The listing builds one solid part. Answer for the finished solid, in the listing's coordinates (mm). A direction names the side the tool comes from. Coordinates: 2 decimals unless noted, no trailing zeros. Write each loop counter-clockwise with the first axis right and the second up, starting at its lowest first coordinate (ties: lowest second). Pieces come first, ordered by that corner, then holes. Notation, with made-up numbers: M 39.5,-32 L 55.5,-32 A23 cw 55.5,-17 Z; hole C 53.25,-30.75 d3. An arc over 180 degrees is marked long. Write item = value, one per line. Start each with the question number.
Autodesk Fusion 360 part; units mm, degrees
sketch "sketch_base_outline" plane through (0, 0, 0) normal (0, 0, 1) x (1, 0, 0)
  line L0 (0, 0) -> (100, 0)
  line L1 (100, 0) -> (100, 60)
  line L2 (100, 60) -> (0, 60)
  line L3 (0, 60) -> (0, 0)
extrude "Extrude1" add sketch "sketch_base_outline" along normal blind 10
sketch "sketch_center_pocket" plane through (0, 0, 10) normal (0, 0, 1) x (1, 0, 0)
  line L0 (0, 60) -> (0, 0)
  line L1 (0, 0) -> (100, 0)
  line L2 (100, 0) -> (100, 60)
  line L3 (100, 60) -> (0, 60)
  line L4 (25, 15) -> (75, 15)
  line L5 (75, 15) -> (75, 45)
  line L6 (75, 45) -> (25, 45)
  line L7 (25, 45) -> (25, 15)
extrude "center_pocket" cut sketch "sketch_center_pocket" against normal blind 3
sketch "sketch_bore_hole" plane through (0, 0, 10) normal (0, 0, 1) x (1, 0, 0)
  line L0 (75, 45) -> (25, 45)
  line L1 (25, 45) -> (25, 15)
  line L2 (25, 15) -> (75, 15)
  line L3 (75, 15) -> (75, 45)
  circle A0 centre (18, 18) radius 6
extrude "bore_hole" cut sketch "sketch_bore_hole" against normal blind 10 contours A0
equation "d3 = -( 3 mm )"
equation "d5 = -( 10 mm )"
1. The part is cut by section C-C, the plane x = 73. Write down the section's boundary in (y, z), and give its area (3 significant figures).
2. Straight lines are drawn through the part: L1, parallel to Y at x = 18, z = 5.5; L2, parallel to Z at x = 87.5, y = 12; L3, parallel to Y at x = 33, z = 7.25. For each, find the intervals that lie inside material, in ascending order. Write a range as [from, to].
3. The part is cut by section B-B, the plane z = 5.5. Write down the section's boundary in (x, y).
4. For a pull along Y with two mould halves and no side action, classify faces 1 (the face through (51, 60, 3)), 2 (the face through (75, 30, 9)), 3 (the face through (49, 0, 3)), 4 (the face through (23.54, 15.7, 3.55)) as pulls with the +Y half, pulls with the -Y half, needs draft (parallel to the pull), parting line crosses it, or undercut.
5. The part is cut by section A-A, the plane y = 18. Write down the section's boundary in (x, z), and give its area (3 significant figures).
6. For faces 5 (the face through (49, 30, 0)), 6 (the face through (50, 15, 9)), 7 (the face through (50, 45, 9)), 8 (the face through (25, 30, 9)), determine the directions among +Z, -Z, +X, -X, +Y, -Y from which every point of the face is accessible in a straight line to the end or side of a thin tool.
7. Each of these flat-tipped pins is pushed along its axis until it touches: pin 1 (2.5 mm diameter, centred on x = 41, z = 9, fed in from -Y); pin 2 (9.5 mm diameter, centred on x = 18, y = 18, fed in from -Z); pin 3 (1 mm diameter, centred on x = 47.5, z = 8.5, fed in from +Y); pin 4 (3.5 mm diameter, centred on y = 26, z = 9, fed in from +X). Where does it stop, or does it pass through?
8. The part is cut by section D-D, the plane x = 18. Write down the section's boundary in (y, z), and give its area (3 significant figures).
Solution:
q1.outline = M 0,0 L 60,0 L 60,7 L 45,7 L 45,10 L 15,10 L 15,7 L 0,7 Z
q1.area = 510 mm^2
q2.L1 = [0, 12], [24, 60]
q2.L2 = [0, 7]
q2.L3 = [15, 45]
q3.outline = M 0,0 L 100,0 L 100,60 L 0,60 Z; hole C 18,18 d12
q4.face_1 = pulls with the +Y half
q4.face_2 = needs draft
q4.face_3 = pulls with the -Y half
q4.face_4 = undercut
q5.outline = M 0,0 L 12,0 L 12,7 L 0,7 Z; M 24,0 L 100,0 L 100,7 L 75,7 L 75,10 L 25,10 L 25,7 L 24,7 Z
q5.area = 766 mm^2
q6.face_5 = -Z, +X, -X, +Y, -Y
q6.face_6 = +Z, +X, -X, -Y
q6.face_7 = +Z, +X, -X, +Y
q6.face_8 = +Z, -X, +Y, -Y
q7.pin_1 = 15
q7.pin_2 = through
q7.pin_3 = 45
q7.pin_4 = 75
q8.outline = M 0,0 L 12,0 L 12,7 L 0,7 Z; M 24,0 L 60,0 L 60,7 L 24,7 Z
q8.area = 336 mm^2
